Could you check a few things on this model? Use its own coordinates, in mm. Face numbers are marked on the shaded views. Round coordinates to 2 decimals unless told otherwise and drop trailing zeros. Write each loop counter-clockwise with the first axis right and the second up, starting at its lowest first coordinate (ties: lowest second). Pieces come first, ordered by that corner, then holes. Notation, with made-up numbers: (-5, 25.5) -> (44, 25.5) arc R14 ccw to (44, 29.5) -> close; hole circle Ø5 at (76, 16.5). An arc over 180 degrees is marked (long way). Answer in a Markdown table with one row per item.
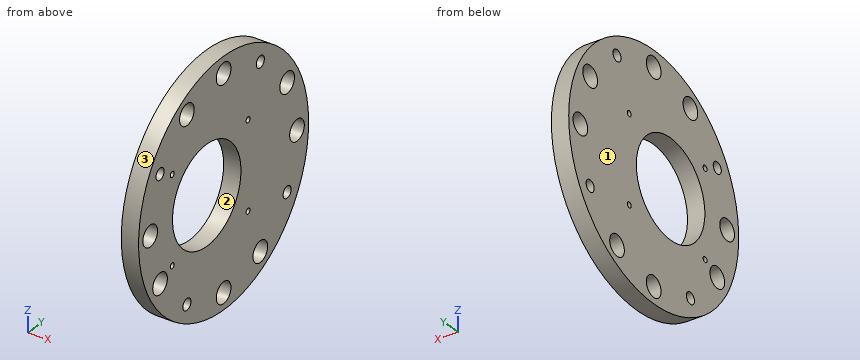
Autodesk Inventor part; units mm, degrees
ref_plane "YZ Plane" through (0, 0, 0) normal (1, 0, 0) x (0, 1, 0)
ref_plane "XZ Plane" through (0, 0, 0) normal (0, 1, 0) x (-1, 0, 0)
ref_plane "XY Plane" through (0, 0, 0) normal (0, 0, 1) x (1, 0, 0)
sketch "Sketch1" plane through (0, 0, 0) normal (1, 0, 0) x (0, 1, 0)
  circle A0 centre (0, 0) radius 34.75
  circle A1 centre (-6.9, 0) radius 14
  dimension "d0" = 69.5
  dimension "d1" = 28
  dimension "d2" = 6.9
extrude "Extrusion1" add sketch "Sketch1" along normal blind 2
sketch "Sketch2" plane through (0, 0, 0) normal (-1, 0, 0) x (0, 0, 1)
  circle A0 centre (0, 0) radius 30
  line L0 (0, 0) -> (25.9808, 15)
  line L1 (0, 0) -> (30, 0) construction
  dimension "d5" = 60
  dimension "d6" = 30
hole "Hole1" at (0, 15, 25.9808) direction (1, 0, 0) diameter 3.3 depth 5
pattern_circular "Circular Pattern1" count 4 over 360 about axis through (0, 0, 0) along (1, 0, 0) of "Hole1"
thread "Thread1"
thread "Thread2"
thread "Thread3"
thread "Thread4"
sketch "Sketch3" plane through (2, 0, 0) normal (1, 0, 0) x (0, 0, -1)
  circle A0 centre (0, 0) radius 30
  point P0 (0, 30)
  dimension "d25" = 60
hole "Hole2" at (2, 30, 0) direction (-1, 0, 0) diameter 6 depth 5
pattern_circular "Circular Pattern2" count 4 over 360 about axis through (0, 0, 0) along (1, 0, 0) of "Hole2"
sketch "Sketch4" plane through (0, 0, 0) normal (-1, 0, 0) x (0, 0, 1)
  circle A0 centre (0, 0) radius 30
  line L0 (0, 0) -> (15, 25.9808)
  line L1 (0, 0) -> (30, 0) construction
  point P0 (15, 25.9808)
  dimension "d36" = 60
  dimension "d37" = 60
hole "Hole3" at (0, 25.9808, 15) direction (1, 0, 0) diameter 6 depth 5
pattern_circular "Circular Pattern3" count 4 over 360 about axis through (0, 0, 0) along (1, 0, 0) of "Hole3"
thicken "Thicken1" operation add thickness 3 both sides no extend neighbours yes toward (-1, 0, 0) faces at (0, 19.5446, -6.1067)
sketch "Sketch5" plane through (-3, 0, 0) normal (-1, 0, 0) x (0, 0, 1)
  line L0 (-12.5, 10) -> (12.5, 10)
  line L1 (12.5, 10) -> (12.5, -21)
  line L2 (12.5, -21) -> (-12.5, -21)
  line L3 (-12.5, -21) -> (-12.5, 10)
  point P0 (0, 0)
  point P1 (0, 10)
  dimension "d50" = 25
  dimension "d51" = 10
  dimension "d52" = 31
hole "Hole4" at (-3, 10, -12.5) at (-3, 10, 12.5) at (-3, -21, 12.5) at (-3, -21, -12.5) direction (1, 0, 0) diameter 1.6 depth 5
thread "Thread5"
thread "Thread6"
thread "Thread7"
thread "Thread8"
properties part number "sample-transfer_adapter-plate"
1) For pin 1 (2 mm diameter, centred on y = -15, z = -25.98, fed in from -X); pin 2 (2 mm diameter, centred on x = 0.5, z = -21.5, fed in from +Y); pin 3 (2 mm diameter, centred on x = 0.5, z = 13, fed in from +Y), each with a flat end and sliding along its axis, tell me the tip position at first contact or that it passes through.
Findings:
| item | result |
|---|---|
| pin 1 | passes through |
| pin 2 | stops at y = 28.06 |
| pin 3 | stops at y = 32.61 |
2) Imagine slicing it at B-B, the plane y = 30. Please give me the cut outline in (x, z), plus the area to 3 significant figures.
Findings:
| item | result |
|---|---|
| outline | (-3, -17.54) -> (2, -17.54) -> (2, -3) -> (-3, -3) -> close; (-3, 3) -> (2, 3) -> (2, 17.54) -> (-3, 17.54) -> close |
| area | 145 mm^2 |
3) Imagine slicing it at C-C, the plane z = 15. Please give me the cut outline in (x, y), plus the area to 3 significant figures.
Findings:
| item | result |
|---|---|
| outline | (-3, -31.35) -> (2, -31.35) -> (2, -27.63) -> (-3, -27.63) -> close; (-3, -24.33) -> (2, -24.33) -> (2, 22.98) -> (-3, 22.98) -> close; (-3, 28.98) -> (2, 28.98) -> (2, 31.35) -> (-3, 31.35) -> close |
| area | 267 mm^2 |
4) Imagine slicing it at D-D, the plane x = -1.55. Count the separate pieces of the cut face and the enclosed holes in it, plus the area to 3 significant figures.
Findings:
| item | result |
|---|---|
| separate pieces | 1 |
| enclosed holes | 17 |
| area | 2,910 mm^2 |
5) Imagine slicing it at A-A, the plane z = 0. Please give me the cut outline in (x, y), plus the area to 4 significant figures.
Findings:
| item | result |
|---|---|
| outline | (-3, -34.75) -> (2, -34.75) -> (2, -33) -> (-3, -33) -> close; (-3, -27) -> (2, -27) -> (2, -20.9) -> (-3, -20.9) -> close; (-3, 7.1) -> (2, 7.1) -> (2, 27) -> (-3, 27) -> close; (-3, 33) -> (2, 33) -> (2, 34.75) -> (-3, 34.75) -> close |
| area | 147.5 mm^2 |
6) Please list where these lines run through material, in increasing order: line 1 (Y direction, x = -1.85, z = -12.5); line 2 (Y direction, x = -1.85, z = 15); line 3 (Z direction, x = -2.2, y = 15.5).
Findings:
| item | result |
|---|---|
| line 1 | y = -32.42 to -27.64, -24.32 to -21.8, -20.2 to -13.2, -0.6 to 9.2, 10.8 to 32.42 |
| line 2 | y = -31.35 to -27.63, -24.33 to 22.98, 28.98 to 31.35 |
| line 3 | z = -31.1 to -28.94, -23.02 to 24.41, 27.55 to 31.1 |
7) Thinking about a two-plate mould opening in Z: for the marked faces 1, 2 and 3, which applies, +Z half, -Z half, draft (parallel to the pull), parting line (faces both ways), or undercut?
Findings:
| item | result |
|---|---|
| face 1 | draft |
| face 2 | undercut |
| face 3 | parting line |
